```python
from build123d import *

# Parameters (mm, degrees)
BOSS_EXTRUDE1_DEPTH     = 254.788
SKETCH3_W               = 20
SKETCH3_H               = 20
CUT_EXTRUDE1_DEPTH      = 1040.5
CUT_EXTRUDE4_DEPTH      = 258.211828935
CUT_EXTRUDE4_DEPTH_BACK = 258.211828935
CUT_EXTRUDE8_DEPTH      = 258.211828935
CUT_EXTRUDE8_DEPTH_BACK = 258.211828935


with BuildPart() as part:
    # Sketch1 → Boss-Extrude1 (new body)
    with BuildSketch(Plane(origin=(0, 0, 0), x_dir=(1, 0, 0), z_dir=(0, 1, 0))):
        with BuildLine():
            Line((2.8, 0), (22.8, 0))
            ThreePointArc((22.8, 0), (24.779898987, -0.820101013), (25.6, -2.8))
            Line((25.6, -2.8), (25.6, -22.8))
            ThreePointArc((25.6, -22.8), (24.779898987, -24.779898987), (22.8, -25.6))
            Line((22.8, -25.6), (2.8, -25.6))
            ThreePointArc((2.8, -25.6), (0.820101013, -24.779898987), (0, -22.8))
            Line((0, -22.8), (0, -2.8))
            ThreePointArc((0, -2.8), (0.820101013, -0.820101013), (2.8, 0))
        make_face()
    extrude(amount=BOSS_EXTRUDE1_DEPTH)

    # Sketch3 → Cut-Extrude1 (cut)
    with BuildSketch(Plane(origin=(0, 0, 0), x_dir=(-1, 0, 0), z_dir=(0, -1, 0))):
        with Locations((-12.8, -12.8)):
            Rectangle(SKETCH3_W, SKETCH3_H)
    extrude(amount=-CUT_EXTRUDE1_DEPTH, mode=Mode.SUBTRACT)

    # Sketch4 → Cut-Extrude4 (cut, two sides: drawn at the far end of the back side and taken through both)
    with BuildSketch(Plane.ZY.offset(-1.4).offset(-CUT_EXTRUDE4_DEPTH_BACK)):
        Polygon((-369.209949856, -369.209949856), (0, 0), (26.086303166, 26.086303166), (395.296253022, 395.296253022), (1133.716152734, -343.123646689), (369.209949856, -1107.629849567), align=None)
    extrude(amount=CUT_EXTRUDE4_DEPTH + CUT_EXTRUDE4_DEPTH_BACK, mode=Mode.SUBTRACT)

    # Sketch5 → Cut-Extrude8 (cut, two sides: drawn at the far end of the back side and taken through both)
    with BuildSketch(Plane.ZY.offset(-1.4).offset(-CUT_EXTRUDE8_DEPTH_BACK)):
        Polygon((-369.209949856, 623.997949856), (0, 254.788), (25.6, 229.188), (394.809949856, -140.021949856), (1133.229849567, 598.397949856), (369.209949856, 1362.417849567), align=None)
    extrude(amount=CUT_EXTRUDE8_DEPTH + CUT_EXTRUDE8_DEPTH_BACK, mode=Mode.SUBTRACT)


solid = part.part
```
Source: CAD feature listing. Evaluate the final solid. Frame: model axes, mm. A direction names the side the tool comes from. Coordinates: 2 decimals unless noted, no trailing zeros. Write each loop counter-clockwise with the first axis right and the second up, starting at its lowest first coordinate (ties: lowest second). Pieces come first, ordered by that corner, then holes. Notation, with made-up numbers: M 37.5,80 L 82.5,80 A11 cw 82.5,92 Z; hole C -30.5,4.5 d9. An arc over 180 degrees is marked long. Answer as a JSON object with one key per item and string values.
1. Cut plane A-A on x = 18.5. Output: boundary loops of the cut face in (y, z).
Evaluation:
{"outline": "M 0,0 L 254.79,0 L 251.99,2.8 L 2.8,2.8 Z; M 22.8,22.8 L 231.99,22.8 L 229.19,25.6 L 25.6,25.6 Z"}
2. Draft query along X for faces 3 (the flat face through (22.8, 126, 13)), 4 (the flat face through (13, 126, 25.6)), 5 (the flat face through (0, 126, 13)), 6 (the flat face through (13, 126, 22.8)). Return one class per face: released by +X, released by -X, zero draft, split by the parting line, or undercut.
Evaluation:
{"face 3": "undercut", "face 4": "zero draft", "face 5": "released by -X", "face 6": "undercut"}
3. Contact query for a flat-ended pin moving along its axis: P1, Ø10, axis at x = 4.5, z = 16.5, coming from the +Y side. Output: stop coordinate, or through.
Evaluation:
{"P1": "y = 242.99"}
4. Access query for faces 1 (the flat face through (13, 126, 2.8)), 2 (the flat face through (2, 13, 13)). Directions: +Z, -Z, +X, -X, +Y, -Y. A direction counts if a zero-diameter tool reaches every point of the face in a straight line with its end or side. Return the directions, or none.
Evaluation:
{"face 1": "+Y, -Y", "face 2": "+Z, +X, -X, -Y"}
5. Ray query, L1, parallel to X at y = 52.5, z = 6; L2, parallel to Z at x = 3, y = 239. Return the intervals inside material, ascending.
Evaluation:
{"L1": "0 to 2.8, 22.8 to 25.6", "L2": "0 to 2.8"}
6. Cut plane C-C on z = 11.25. Output: boundary loops of the cut face in (x, y).
Evaluation:
{"outline": "M 0,11.25 L 2.8,11.25 L 2.8,243.54 L 0,243.54 Z; M 22.8,11.25 L 25.6,11.25 L 25.6,243.54 L 22.8,243.54 Z"}
7. Cut plane B-B on y = 102. Output: boundary loops of the cut face in (x, z), plus the area to 3 significant figures.
Evaluation:
{"outline": "M 0,2.8 A2.8 ccw 2.8,0 L 22.8,0 A2.8 ccw 25.6,2.8 L 25.6,22.8 A2.8 ccw 22.8,25.6 L 2.8,25.6 A2.8 ccw 0,22.8 Z; hole M 2.8,2.8 L 22.8,2.8 L 22.8,22.8 L 2.8,22.8 Z", "area": "249 mm^2"}
